Design review of the part built by this model. Coordinates are the model's own, in mm. A direction names the side the tool comes from. Round coordinates to 2 decimals unless told otherwise and drop trailing zeros. Order: outer loops, then holes, each group sorted by start corner. A loop starts at its lowest first (then second) coordinate and runs counter-clockwise, first axis right, second up.
from build123d import *

# Parameters (mm, degrees)
F0_W     = 19.05
F0_H     = 53.34
F0_R     = 2.5527
F1_DEPTH = 5.842
F2_SIZE  = 6.35
F3_SIZE  = 1.524


with BuildPart() as f1:
    # F0 (on Top) → F1 (new body)
    with BuildSketch(Plane.XY):
        with Locations((9.525, -26.67)):
            Rectangle(F0_W, F0_H)
        with BuildLine():
            Line((6.223, -45.2755), (6.223, -16.3195))
            ThreePointArc((6.223, -16.3195), (7.190133, -13.984633), (9.525, -13.0175))
            ThreePointArc((9.525, -13.0175), (11.859867, -13.984633), (12.827, -16.3195))
            Line((12.827, -16.3195), (12.827, -45.2755))
            ThreePointArc((12.827, -45.2755), (11.859867, -47.610367), (9.525, -48.5775))
            ThreePointArc((9.525, -48.5775), (7.190133, -47.610367), (6.223, -45.2755))
        make_face(mode=Mode.SUBTRACT)
        with Locations((9.525, -6.35)):
            Circle(F0_R, mode=Mode.SUBTRACT)
    extrude(amount=F1_DEPTH)

    # F2
    f2_edges = [f1.edges().sort_by_distance(p)[0] for p in [
        (0, -53.34, 2.921),
        (19.05, -53.34, 2.921),
    ]]
    chamfer(f2_edges, length=F2_SIZE)

    # F3
    f3_edges = [f1.edges().sort_by_distance(p)[0] for p in [
        (19.05, 0, 2.921),
        (0, 0, 2.921),
    ]]
    chamfer(f3_edges, length=F3_SIZE)


solid = f1.part
1) Take a section at C-C on x = 11.5. Give the boundary of the cut face in (y, z), plus the area to 3 significant figures.
Results:
outline: (-53.34, 0) - (-47.92, 0) - (-47.92, 5.84) - (-53.34, 5.84) - close; (-13.67, 0) - (-7.97, 0) - (-7.97, 5.84) - (-13.67, 5.84) - close; (-4.73, 0) - (0, 0) - (0, 5.84) - (-4.73, 5.84) - close
area: 92.6 mm2
2) Take a section at A-A on z = 4. State how many separate pieces and enclosed holes the cut face has, plus the area to 3 significant figures.
Results:
separate pieces: 1
enclosed holes: 2
area: 728 mm2
3) Take a section at B-B on y = -42.5. Give the boundary of the cut face in (x, z).
Results:
outline: (0, 0) - (6.22, 0) - (6.22, 5.84) - (0, 5.84) - close; (12.83, 0) - (19.05, 0) - (19.05, 5.84) - (12.83, 5.84) - close
4) The part is to be moulded in two halves that separate along X. For faces 3 (the face through (9, -53.34, 3)), 4 (the face through (18.299, -0.773, 2.88)), 5 (the face through (12.827, -31, 3)), say which applies: released by +X, released by -X, zero draft, split by the parting line, or undercut.
Results:
face 3: zero draft
face 4: released by +X
face 5: undercut
5) To check wall thickness, follow line 1 along Y through (x, z) = (9.5, 4.8); line 2 along X through (y, z) = (-32, 2.4); line 3 along Y through (x, z) = (11.25, 2). State the ranges of each line that lie inside material, in increasing order.
Results:
line 1: y = -53.34 to -48.58, -13.02 to -8.9, -3.8 to 0
line 2: x = 0 to 6.22, 12.83 to 19.05
line 3: y = -53.34 to -48.09, -13.5 to -8.23, -4.47 to 0
6) Take a section at D-D on y = -6.35. Give the boundary of the cut face in (x, z), plus the area to 3 significant figures.
Results:
outline: (0, 0) - (6.97, 0) - (6.97, 5.84) - (0, 5.84) - close; (12.08, 0) - (19.05, 0) - (19.05, 5.84) - (12.08, 5.84) - close
area: 81.5 mm2
7) For faces 1 (the face through (6.223, -31, 3)), 2 (the face through (15.92, -50.12, 2.88)), list the 3-axis set-ups (+Z, -Z, +X, -X, +Y, -Y) from which the entire face can be reached by the end or side of a thin tool; tool diameter is ignored.
Results:
face 1: +Z, -Z
face 2: +Z, -Z, +X, -Y
